Input: part model. Units: mm. Frame: model coordinates. A direction names the side the tool comes from. Give positions to 0.01 mm unless a question says otherwise; leave off trailing zeros. Write each loop counter-clockwise with the first axis right and the second up, starting at its lowest first coordinate (ties: lowest second). Pieces come first, ordered by that corner, then holes. Notation, with made-up numbers: (2, 52.5) - (18, 52.5) arc R24 ccw to (18, 63.5) - close; hole circle Ø2 at (88, 76.5). An arc over 180 degrees is marked (long way). Answer as a JSON object with one key per item and string values. Group by question number.
from build123d import *

# Parameters (mm, degrees)
BOSS_EXTRUDE1_DEPTH = 2
BOSS_EXTRUDE2_START = 3
BOSS_EXTRUDE2_DEPTH = 3
FILLET1_R           = 3


with BuildPart() as part:
    # Sketch1 → Boss-Extrude1 (new body)
    with BuildSketch(Plane.ZY.offset(329.974562358)):
        with BuildLine():
            Line((137.105001839, 14.690261729), (137.105001839, -0.019509128))
            Line((137.105001839, -0.019509128), (133.705001839, -0.019509128))
            Line((133.705001839, -0.019509128), (129.505001839, -0.019509128))
            Line((129.505001839, -0.019509128), (129.505001839, -16.302112125))
            Line((129.505001839, -16.302112125), (-21.848970599, -16.302112125))
            Line((-21.848970599, -16.302112125), (-21.848970599, -0.019509128))
            Line((-21.848970599, -0.019509128), (-26.048970599, -0.019509128))
            Line((-26.048970599, -0.019509128), (-29.448970599, -0.019509128))
            Line((-29.448970599, -0.019509128), (-29.448970599, 47.708117707))
            ThreePointArc((-29.448970599, 47.708117707), (-28.460366767, 49.843262649), (-26.192653512, 50.470684397))
            Line((-26.192653512, 50.470684397), (74.05116687, 33.912543624))
            Line((74.05116687, 33.912543624), (79.277875997, 26.617509644))
            Line((79.277875997, 26.617509644), (134.761318926, 17.452828418))
            ThreePointArc((134.761318926, 17.452828418), (136.440146781, 16.501657897), (137.105001839, 14.690261729))
        make_face()
    extrude(amount=-BOSS_EXTRUDE1_DEPTH)

    # Sketch1<4> → Boss-Extrude2 (add)
    # profile 1 of 3: a face of its own
    with BuildSketch(Plane.ZY.offset(329.974562358).offset(BOSS_EXTRUDE2_START)):
        with BuildLine():
            Line((-32.648970599, -19.502112125), (140.305001839, -19.502112125))
            Line((140.305001839, -19.502112125), (140.305001839, -10.219509128))
            Line((140.305001839, -10.219509128), (133.705001839, -10.219509128))
            Line((133.705001839, -10.219509128), (133.705001839, -0.219509128))
            Line((133.705001839, -0.219509128), (137.305001839, -0.219509128))
            Line((137.305001839, -0.219509128), (137.305001839, 14.690261729))
            ThreePointArc((137.305001839, 14.690261729), (136.592657134, 16.631043337), (134.793913004, 17.650154611))
            Line((134.793913004, 17.650154611), (79.39220526, 26.801334927))
            Line((79.39220526, 26.801334927), (74.165496133, 34.096368907))
            Line((74.165496133, 34.096368907), (-26.160059434, 50.668010589))
            ThreePointArc((-26.160059434, 50.668010589), (-28.589752208, 49.995773002), (-29.648970599, 47.708117707))
            Line((-29.648970599, 47.708117707), (-29.648970599, -0.219509128))
            Line((-29.648970599, -0.219509128), (-26.048970599, -0.219509128))
            Line((-26.048970599, -0.219509128), (-26.048970599, -10.219509128))
            Line((-26.048970599, -10.219509128), (-32.648970599, -10.219509128))
            Line((-32.648970599, -10.219509128), (-32.648970599, -19.502112125))
        make_face()
        with BuildLine():
            ThreePointArc((137.105001839, 14.690261729), (136.440146781, 16.501657897), (134.761318926, 17.452828418))
            Line((134.761318926, 17.452828418), (79.277875997, 26.617509644))
            Line((79.277875997, 26.617509644), (74.05116687, 33.912543624))
            Line((74.05116687, 33.912543624), (-26.192653512, 50.470684397))
            ThreePointArc((-26.192653512, 50.470684397), (-28.460366767, 49.843262649), (-29.448970599, 47.708117707))
            Line((-29.448970599, 47.708117707), (-29.448970599, -0.019509128))
            Line((-29.448970599, -0.019509128), (-26.048970599, -0.019509128))
            Line((-26.048970599, -0.019509128), (-21.848970599, -0.019509128))
            Line((-21.848970599, -0.019509128), (-21.848970599, -16.302112125))
            Line((-21.848970599, -16.302112125), (129.505001839, -16.302112125))
            Line((129.505001839, -16.302112125), (129.505001839, -0.019509128))
            Line((129.505001839, -0.019509128), (133.705001839, -0.019509128))
            Line((133.705001839, -0.019509128), (137.105001839, -0.019509128))
            Line((137.105001839, -0.019509128), (137.105001839, 14.690261729))
        make_face(mode=Mode.SUBTRACT)
    # profile 2 of 3: a face of its own
    with BuildSketch(Plane.ZY.offset(329.974562358).offset(BOSS_EXTRUDE2_START)):
        with BuildLine():
            ThreePointArc((76.604168861, 35.843616835), (75.749893119, 36.643855156), (74.654407298, 37.056261789))
            Line((74.654407298, 37.056261789), (-29.160059434, 54.204197172))
            ThreePointArc((-29.160059434, 54.204197172), (-31.589752208, 53.531959584), (-32.648970599, 51.24430429))
            Line((-32.648970599, 51.24430429), (-32.648970599, -10.219509128))
            Line((-32.648970599, -10.219509128), (-26.048970599, -10.219509128))
            Line((-26.048970599, -10.219509128), (-26.048970599, -0.219509128))
            Line((-26.048970599, -0.219509128), (-29.648970599, -0.219509128))
            Line((-29.648970599, -0.219509128), (-29.648970599, 47.708117707))
            ThreePointArc((-29.648970599, 47.708117707), (-28.589752208, 49.995773002), (-26.160059434, 50.668010589))
            Line((-26.160059434, 50.668010589), (74.165496133, 34.096368907))
            Line((74.165496133, 34.096368907), (79.39220526, 26.801334927))
            Line((79.39220526, 26.801334927), (134.793913004, 17.650154611))
            ThreePointArc((134.793913004, 17.650154611), (136.592657134, 16.631043337), (137.305001839, 14.690261729))
            Line((137.305001839, 14.690261729), (137.305001839, -0.219509128))
            Line((137.305001839, -0.219509128), (133.705001839, -0.219509128))
            Line((133.705001839, -0.219509128), (133.705001839, -10.219509128))
            Line((133.705001839, -10.219509128), (140.305001839, -10.219509128))
            Line((140.305001839, -10.219509128), (140.305001839, 17.2353763))
            ThreePointArc((140.305001839, 17.2353763), (139.592657134, 19.176157909), (137.793913004, 20.195269182))
            Line((137.793913004, 20.195269182), (82.333171975, 29.356200538))
            ThreePointArc((82.333171975, 29.356200538), (81.237686153, 29.768607171), (80.383410411, 30.568845492))
            Line((80.383410411, 30.568845492), (76.604168861, 35.843616835))
        make_face()
    # profile 3 of 3: a face of its own
    with BuildSketch(Plane.ZY.offset(329.974562358).offset(BOSS_EXTRUDE2_START)):
        with BuildLine():
            Line((137.105001839, 14.690261729), (137.105001839, -0.019509128))
            Line((137.105001839, -0.019509128), (133.705001839, -0.019509128))
            Line((133.705001839, -0.019509128), (129.505001839, -0.019509128))
            Line((129.505001839, -0.019509128), (129.505001839, -16.302112125))
            Line((129.505001839, -16.302112125), (-21.848970599, -16.302112125))
            Line((-21.848970599, -16.302112125), (-21.848970599, -0.019509128))
            Line((-21.848970599, -0.019509128), (-26.048970599, -0.019509128))
            Line((-26.048970599, -0.019509128), (-29.448970599, -0.019509128))
            Line((-29.448970599, -0.019509128), (-29.448970599, 47.708117707))
            ThreePointArc((-29.448970599, 47.708117707), (-28.460366767, 49.843262649), (-26.192653512, 50.470684397))
            Line((-26.192653512, 50.470684397), (74.05116687, 33.912543624))
            Line((74.05116687, 33.912543624), (79.277875997, 26.617509644))
            Line((79.277875997, 26.617509644), (134.761318926, 17.452828418))
            ThreePointArc((134.761318926, 17.452828418), (136.440146781, 16.501657897), (137.105001839, 14.690261729))
        make_face()
    extrude(amount=-BOSS_EXTRUDE2_DEPTH)

    # Fillet1
    fillet1_edges = [part.edges().sort_by_distance(p)[0] for p in [
        (-332.974562358, 15.871096082, -32.648970599),
        (-332.974562358, 53.531959584, -31.589752208),
        (-332.974562358, 45.63022948, 22.747173932),
        (-332.974562358, 36.643855156, 75.749893119),
        (-332.974562358, 33.206231163, 78.493789636),
        (-332.974562358, 29.768607171, 81.237686153),
        (-332.974562358, 24.77573486, 110.063542489),
        (-332.974562358, 19.176157909, 139.592657134),
        (-332.974562358, -1.133367912, 140.305001839),
    ]]
    fillet(fillet1_edges, radius=FILLET1_R - 0.0001)  # a hair under: the kernel refuses the full size


with BuildPart() as body_2:
    # Mirror1: mirrored copy
    add(part.part.mirror(Plane.ZY.offset(327.974562358)))


solid = part.part
1) Pin query (flat end, axial travel): P1, Ø3, axis at x = -330, z = 106.5, coming from the +Y side; P2, Ø1, axis at x = -329, z = 83.5, coming from the -Y side; P3, Ø0.6, axis at x = -329.5, y = -6, coming from the -Z side. Return the tip coordinate at first contact, or that it passes through.
2) Line query: line 1 along Z through (x, y) = (-329.55, -11.5) (3 decimals); line 2 along Z through (x, y) = (-328.85, 7) (3 decimals); line 3 along X through (y, z) = (-10.5, -25). Output: solid intervals per line, ascending. Write a range as from..to.
3) Cut plane B-B on x = -328.95. Return the cut outline in (y, z) (1 decimal), and give its area (3 significant figures).
4) Reachability of faces 1 (the face through (-328.989, 42.308, 23.228)), 2 (the face through (-332.119, 16.366, -31.747)) from +Z, -Z, +X, -X, +Y, -Y: full face, straight path, thin tool, end or side. Return the list, or none.
Filled in:
{
 "1": {"P1": "stops at y = 25.61", "P2": "stops at y = -16.3", "P3": "stops at z = -21.85"},
 "2": {"line 1": "z = -21.849..129.505", "line 2": "z = -29.449..137.105", "line 3": "x = -332.97..-329.97"},
 "3": {"outline": "(-16.3, -21.8) - (0, -21.8) - (0, -29.4) - (47.7, -29.4) arc R2.8 ccw to (50.5, -26.2) - (33.9, 74.1) - (26.6, 79.3) - (17.5, 134.8) arc R2.8 ccw to (14.7, 137.1) - (0, 137.1) - (0, 129.5) - (-16.3, 129.5) - close", "area": "8,280 mm²"},
 "4": {"face 1": "+Z, +X, +Y", "face 2": "-Z, -X, +Y, -Y"}
}
